Here's how the part is built. I have some questions about the finished solid (model axes, mm). Face numbers are marked on the shaded views. A direction names the side the tool comes from. Give positions to 0.01 mm unless a question says otherwise; leave off trailing zeros. Loops run counter-clockwise (first coordinate to the right, second up) from the corner with the lowest first, then second, coordinate; pieces in that order, holes last.
Q1. Suppose I cut it at C-C (z = 23). List the corners of the cut face in (x, y) for me (3 decimals), and give its area (3 significant figures).
Q2. I'm going to push flat-ended pins straight in: P1, Ø1, axis at x = 24, y = 7.5, coming from the -Z side; P2, Ø2, axis at x = -29.5, z = 27, coming from the +Y side; P3, Ø20, axis at x = -4, y = -5, coming from the -Z side; P4, Ø3, axis at y = 14, z = 24, coming from the -X side. Where does each tip first touch, or does it pass through?
Q3. Suppose I cut it at A-A (x = -50.8). List the corners of the cut face in (y, z) for me (3 decimals).
Q4. Suppose I cut it at D-D (y = 0). Count the separate pieces of the cut face and the enclosed holes in it, and give its area (3 significant figures).
Q5. Thinking about a two-plate mould opening in X: for the marked faces 4, 5 and 6, which applies, pulls with the +X half, pulls with the -X half, needs draft (parallel to the pull), parting line crosses it, or undercut?
Q6. I need wall thicknesses on probe 1 along Y at (x, z) = (0, 37.7) (3 decimals); probe 2 along Y at (x, z) = (50.8, 0.55) (3 decimals); probe 3 along Z at (x, y) = (-51, -11.5). Which ranges of each line are inside material? Lowest first, please.
Q7. Suppose I cut it at B-B (x = 0). List the corners of the cut face in (y, z) for me (3 decimals).
Q8. For the marked faces 1, 2 and 3, which set-ups out of +Z, -Z, +X, -X, +Y, -Y let a thin tool reach every point of the face, with its end or its side?
```python
from build123d import *

# Parameters (mm, degrees)
BASE_FLANGE1_DEPTH                    = 22.225
F_28_0_1405_DIAMETER_HOLE1_AT_2_COUNT = 2
F_28_0_1405_DIAMETER_HOLE1_AT_2_PITCH = 101.6
F_19_0_166_DIAMETER_HOLE1_D           = 4.2164


# Sheet-metal steps are written as plain solids
with BuildPart() as part:
    # Sketch2 → Base-Flange1 (new, symmetric)
    with BuildSketch(Plane(origin=(0, 0, 0), x_dir=(1, 0, 0), z_dir=(0, 1, 0))):
        with BuildLine():
            Line((60.325, 0), (42.418846353, 0))
            ThreePointArc((42.418846353, 0), (41.428246353, -0.26543047), (40.703076823, -0.9906))
            Line((40.703076823, -0.9906), (20.311815871, -36.3093))
            ThreePointArc((20.311815871, -36.3093), (20.172360192, -36.448755679), (19.981860192, -36.4998))
            Line((19.981860192, -36.4998), (-19.981860192, -36.4998))
            ThreePointArc((-19.981860192, -36.4998), (-20.172360192, -36.448755679), (-20.311815871, -36.3093))
            Line((-20.311815871, -36.3093), (-40.703076823, -0.9906))
            ThreePointArc((-40.703076823, -0.9906), (-41.428246353, -0.26543047), (-42.418846353, 0))
            Line((-42.418846353, 0), (-60.325, 0))
            Line((-60.325, 0), (-60.325, -1.6002))
            Line((-60.325, -1.6002), (-42.418846353, -1.6002))
            ThreePointArc((-42.418846353, -1.6002), (-42.228346353, -1.651244321), (-42.088890674, -1.7907))
            Line((-42.088890674, -1.7907), (-21.697629722, -37.1094))
            ThreePointArc((-21.697629722, -37.1094), (-20.972460192, -37.83456953), (-19.981860192, -38.1))
            Line((-19.981860192, -38.1), (19.981860192, -38.1))
            ThreePointArc((19.981860192, -38.1), (20.972460192, -37.83456953), (21.697629722, -37.1094))
            Line((21.697629722, -37.1094), (42.088890674, -1.7907))
            ThreePointArc((42.088890674, -1.7907), (42.228346353, -1.651244321), (42.418846353, -1.6002))
            Line((42.418846353, -1.6002), (60.325, -1.6002))
            Line((60.325, -1.6002), (60.325, 0))
        make_face()
    extrude(amount=BASE_FLANGE1_DEPTH, both=True)

    # Sketch4 → #28 (0.1405) Diameter Hole1 (revolve, cut)
    with BuildSketch(Plane(origin=(50.8, 0, 1.6002), x_dir=(0, -1, 0), z_dir=(1, 0, 0))):
        Polygon((0, 0), (0, 1.6002), (1.9812, 1.6002), (1.78435, 1.40335), (1.78435, 0.19685), (1.9812, 0), align=None)
    f_28_0_1405_diameter_hole1 = revolve(axis=Axis((50.8, 0, 7.9502), (0, 0, -1)), mode=Mode.SUBTRACT)

    # #28 (0.1405) Diameter Hole1 at 2: #28 (0.1405) Diameter Hole1 ×2
    with Locations(*[(-i * F_28_0_1405_DIAMETER_HOLE1_AT_2_PITCH, 0, 0) for i in range(1, F_28_0_1405_DIAMETER_HOLE1_AT_2_COUNT)]):
        add(f_28_0_1405_diameter_hole1, mode=Mode.SUBTRACT)

    # #19 (0.166) Diameter Hole1 (through all)
    with Locations(Plane.XY.offset(38.1)):
        with Locations((0, 5.9944), (0, -5.9944)):
            Hole(F_19_0_166_DIAMETER_HOLE1_D / 2)


solid = part.part
```
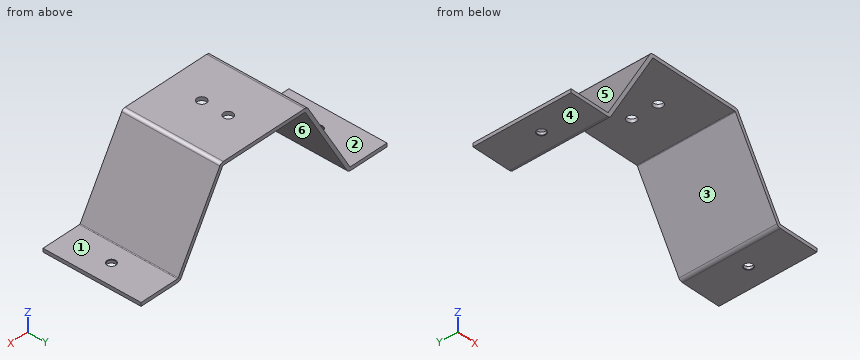
Solutions:
1. outline: (-29.844, -22.225) - (-27.996, -22.225) - (-27.996, 22.225) - (-29.844, 22.225) - close; (27.996, -22.225) - (29.844, -22.225) - (29.844, 22.225) - (27.996, 22.225) - close
1. area: 164 mm2
2. P1: stops at z = 29.06
2. P2: passes through
2. P3: stops at z = 36.5
2. P4: stops at x = -30.13
3. outline: (-22.225, 0) - (-1.981, 0) - (-1.784, 0.197) - (-1.784, 1.403) - (-1.981, 1.6) - (-22.225, 1.6) - close; (1.784, 0.197) - (1.981, 0) - (22.225, 0) - (22.225, 1.6) - (1.981, 1.6) - (1.784, 1.403) - close
4. separate pieces: 3
4. enclosed holes: 0
4. area: 248 mm2
5. face 4: needs draft
5. face 5: pulls with the -X half
5. face 6: undercut
6. probe 1: y = -22.225 to -8.103, -3.886 to 3.886, 8.103 to 22.225
6. probe 2: y = -22.225 to -1.784, 1.784 to 22.225
6. probe 3: z = 0 to 1.6
7. outline: (-22.225, 36.5) - (-8.103, 36.5) - (-8.103, 38.1) - (-22.225, 38.1) - close; (-3.886, 36.5) - (3.886, 36.5) - (3.886, 38.1) - (-3.886, 38.1) - close; (8.103, 36.5) - (22.225, 36.5) - (22.225, 38.1) - (8.103, 38.1) - close
8. face 1: +Z, +X, +Y, -Y
8. face 2: +Z, -X, +Y, -Y
8. face 3: -Z, +Y, -Y
